```python
from build123d import *

# Parameters (mm, degrees)
BOSS_EXTRUDE1_DEPTH = 2
SKETCH1_3_R         = 1
BOSS_EXTRUDE2_DEPTH = 5


with BuildPart() as part:
    # Sketch1 → Boss-Extrude1 (new body)
    with BuildSketch(Plane.XY):
        with BuildLine():
            Line((-0.025909327, -13.500223781), (55.727261904, -12.537061992))
            ThreePointArc((55.727261904, -12.537061992), (57.25294745, -14.010928883), (55.779080559, -15.536614429))
            Line((55.779080559, -15.536614429), (0.025909327, -16.499776219))
            ThreePointArc((0.025909327, -16.499776219), (-1.499776219, -15.025909327), (-0.025909327, -13.500223781))
        make_face()
    extrude(amount=BOSS_EXTRUDE1_DEPTH)

    # Sketch1<3> → Boss-Extrude2 (add)
    with BuildSketch(Plane.XY):
        with Locations((0, -15)):
            Circle(SKETCH1_3_R)
        with Locations((55.753171232, -14.03683821)):
            Circle(SKETCH1_3_R)
    extrude(amount=-BOSS_EXTRUDE2_DEPTH)


solid = part.part
```
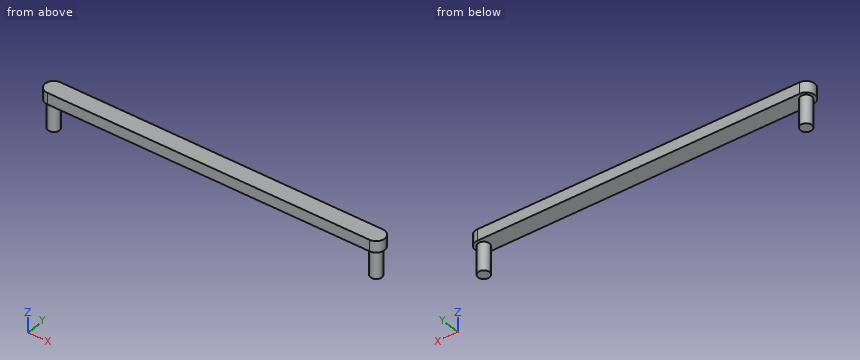
Here's how the part is built. I have some questions about the finished solid (model axes, mm). Round coordinates to 2 decimals unless told otherwise and drop trailing zeros. Loops run counter-clockwise (first coordinate to the right, second up) from the corner with the lowest first, then second, coordinate; pieces in that order, holes last. Notation, with made-up numbers: (-13, -3) -> (10, -3) arc R16 cw to (10, 10) -> close; hole circle Ø11 at (58, 54). An arc over 180 degrees is marked (long way). Answer as CSV lines item,"result". Start each with the question number.
1. I'm going to push flat-ended pins straight in: P1, Ø1, axis at x = 18.5, y = -14, coming from the -Z side; P2, Ø4, axis at x = 38.5, z = -1.5, coming from the -Y side; P3, Ø3, axis at x = 28, z = -1, coming from the -Y side. Where does each tip first touch, or does it pass through?
2. Imagine slicing it at A-A on z = 0.5. Write out the boundary of the cut face in (x, y), plus the area to 3 significant figures.
3. Imagine slicing it at B-B on x = 23. Write out the boundary of the cut face in (y, z).
4. I need wall thicknesses on probe 1 along Z at (x, y) = (45, -14.35); probe 2 along X at (y, z) = (-13.95, -1.5); probe 3 along X at (y, z) = (-14.75, -1.25). Which ranges of each line are inside material? Lowest first, please. Write a range as from..to.
Solution:
1,P1,"z = 0"
1,P2,"y = -15.86"
1,P3,"y = -16.04"
2,outline,"(-0.03, -13.5) arc R1.5 ccw to (0.03, -16.5) -> (55.78, -15.54) arc R1.5 ccw to (55.73, -12.54) -> close"
2,area,"174 mm²"
3,outline,"(-16.1, 0) -> (-13.1, 0) -> (-13.1, 2) -> (-16.1, 2) -> close"
4,probe 1,"0..2"
4,probe 2,"54.76..56.75"
4,probe 3,"-0.97..0.97, 55.05..56.45"
